```python
from build123d import *

# Parameters (mm, degrees)
BOSS_EXTRUDE1_DEPTH     = 1.5
SKETCH7_W               = 3
SKETCH7_H               = 80
BOSS_EXTRUDE2_DEPTH     = 4.655
CHAMFER1_SIZE           = 1.5
CUT_EXTRUDE1_DEPTH      = 83.983432081
CUT_EXTRUDE1_DEPTH_BACK = 83.983432081
SKETCH8_W               = 4.655
SKETCH8_H               = 35


with BuildPart() as part:
    # Sketch1 → Boss-Extrude1 (new, symmetric)
    with BuildSketch(Plane.XY):
        Polygon((0, 0), (0, 80), (22, 10), (22, -10), align=None)
    extrude(amount=BOSS_EXTRUDE1_DEPTH, both=True)

    # Sketch7 → Boss-Extrude2 (add)
    with BuildSketch(Plane.ZY):
        with Locations((0, 40)):
            Rectangle(SKETCH7_W, SKETCH7_H)
    extrude(amount=BOSS_EXTRUDE2_DEPTH)

    # Chamfer1
    chamfer1_edges = [part.edges().sort_by_distance(p)[0] for p in [
        (11, -5, 1.5),
        (11, -5, -1.5),
        (11, 45, -1.5),
        (11, 45, 1.5),
    ]]
    chamfer(chamfer1_edges, length=CHAMFER1_SIZE - 0.0001)  # a hair under: the kernel refuses the full size

    # Sketch8 → Cut-Extrude1 (cut, two sides: drawn at the far end of the back side and taken through both)
    with BuildSketch(Plane.XY.offset(-CUT_EXTRUDE1_DEPTH_BACK)):
        with Locations((-2.3275, 17.5)):
            Rectangle(SKETCH8_W, SKETCH8_H)
    extrude(amount=CUT_EXTRUDE1_DEPTH + CUT_EXTRUDE1_DEPTH_BACK, mode=Mode.SUBTRACT)


solid = part.part
```
Geometry check sheet. Reference: the model listing, model coordinates, mm. A direction names the side the tool comes from. Round coordinates to 2 decimals unless told otherwise and drop trailing zeros. Loops run counter-clockwise (first coordinate to the right, second up) from the corner with the lowest first, then second, coordinate; pieces in that order, holes last. Notation, with made-up numbers: (58.25, -16) -> (112.25, -16) arc R23 ccw to (112.25, 3) -> close; hole circle Ø6 at (67.25, -27.75). An arc over 180 degrees is marked (long way). Use a Markdown table: item, result.
(1) Sectioned sample at C-C (z = 0.9). Enter the section's corners in (x, y) (1 decimal), then the cut area to 3 significant figures.
Calculated:
| item | result |
|---|---|
| outline | (-4.7, 35) -> (0, 35) -> (0, 0) -> (2.2, 0) -> (22, -9) -> (22, 7) -> (-0.9, 80) -> (-4.7, 80) -> close |
| area | 1,220 mm² |
(2) Set-up check for faces 1 (the flat face through (22, -2, 0)), 2 (the flat face through (0, 17, 0)), 3 (the flat face through (1, 0, 1)), 4 (the flat face through (1, 0, -1)): record each of +Z, -Z, +X, -X, +Y, -Y from which the full face is reachable in a straight line by a thin tool's end or side.
Calculated:
| item | result |
|---|---|
| face 1 | +Z, -Z, +X, +Y, -Y |
| face 2 | +Z, -Z, -X, -Y |
| face 3 | +Z, -X, -Y |
| face 4 | -Z, -X, -Y |
(3) Scan lines: probe 1 along X at (y, z) = (4.5, 0.85); probe 2 along Y at (x, z) = (-1.25, 0.5); probe 3 along X at (y, z) = (40, -1) (3 decimals). Record each from-to range of solid material in increasing order.
Calculated:
| item | result |
|---|---|
| probe 1 | 0 to 22 |
| probe 2 | 35 to 80 |
| probe 3 | -4.655 to 11.523 |
(4) Go/stop test with flat-tipped pins: P1, Ø1.5, axis at y = 11.5, z = 0.5, coming from the -X side; P2, Ø0.7, axis at x = 2.5, z = 0.5, coming from the -Y side; P3, Ø1, axis at x = 16.5, z = -1, coming from the -Y side. Record where each tip stops, or that it passes through.
Calculated:
| item | result |
|---|---|
| P1 | x = 0 |
| P2 | y = -1 |
| P3 | y = -7 |
(5) Sectioned sample at B-B (y = 2.5). Enter the section's corners in (x, z).
Calculated:
| item | result |
|---|---|
| outline | (0, -1.5) -> (22, -1.5) -> (22, 1.5) -> (0, 1.5) -> close |
